Can you work these out from the model? Positions are in its coordinate system, mm. Coordinates: 2 decimals unless noted, no trailing zeros. Order: outer loops, then holes, each group sorted by start corner. A loop starts at its lowest first (then second) coordinate and runs counter-clockwise, first axis right, second up. Notation, with made-up numbers: (39, -6.75) -> (93, -6.75) arc R33 cw to (93, 26.25) -> close; hole circle Ø2 at (61.5, -33.5). An arc over 180 degrees is marked (long way). Answer as a JSON object with one key per item and string values. Group by question number.
(1) I want a section at A-A, the plane z = 0. List the corners of the cut face in (x, y) for me.
(2) I need wall thicknesses on line 1 (Y direction, x = 1.3, z = 0.1); line 2 (Y direction, x = 1.3, z = 0.7); line 3 (Z direction, x = -0.95, y = 3). Which ranges of each line are inside material? Lowest first, please.
(3) For pin 1 (1.5 mm diameter, centred on y = 56.5, z = 1, fed in from +X), with a flat end and sliding along its axis, tell me the tip position at first contact or that it passes through.
(4) I want a section at C-C, the plane y = 71.2. List the corners of the cut face in (x, z) for me (1 decimal), plus the area to 3 significant figures.
(5) I want a section at B-B, the plane y = 34.5. List the corners of the cut face in (x, z) for me (1 decimal), plus the area to 3 significant figures.
from build123d import *

# Parameters (mm, degrees)
SKETCH1_R                      = 1.5875
BOSS_EXTRUDE1_DEPTH            = 74.2
CUT_EXTRUDE1_REACH             = 3.587
SKETCH2_R                      = 1
CUT_EXTRUDE1_DIRECTION_2_REACH = 3.587


with BuildPart() as part:
    # Sketch1 → Boss-Extrude1 (new body)
    with BuildSketch(Plane(origin=(0, 0, 0), x_dir=(1, 0, 0), z_dir=(0, 1, 0))):
        Circle(SKETCH1_R)
    extrude(amount=BOSS_EXTRUDE1_DEPTH)

    # Sketch2 → Cut-Extrude1 (cut, up to next)
    with BuildSketch(Plane(origin=(0, 0, 0), x_dir=(0, 0, -1), z_dir=(1, 0, 0)), mode=Mode.PRIVATE) as cut_extrude1_sk1:
        with Locations((0, 71.2)):
            Circle(SKETCH2_R)
    cut_extrude1_tool1 = extrude(cut_extrude1_sk1.sketch, amount=-CUT_EXTRUDE1_REACH, mode=Mode.PRIVATE) & part.part
    add(cut_extrude1_tool1.solids().sort_by_distance((0, 71.2, 0))[0], mode=Mode.SUBTRACT)
    # Sketch2 → Cut-Extrude1 (cut, up to next)
    with BuildSketch(Plane(origin=(0, 0, 0), x_dir=(0, 0, -1), z_dir=(1, 0, 0)), mode=Mode.PRIVATE) as cut_extrude1_sk2:
        with Locations((0, 3)):
            Circle(SKETCH2_R)
    cut_extrude1_tool2 = extrude(cut_extrude1_sk2.sketch, amount=-CUT_EXTRUDE1_REACH, mode=Mode.PRIVATE) & part.part
    add(cut_extrude1_tool2.solids().sort_by_distance((0, 3, 0))[0], mode=Mode.SUBTRACT)

    # Sketch2 → Cut-Extrude1 direction 2 (cut, up to next)
    with BuildSketch(Plane(origin=(0, 0, 0), x_dir=(0, 0, -1), z_dir=(1, 0, 0)), mode=Mode.PRIVATE) as cut_extrude1_direction_2_sk1:
        with Locations((0, 71.2)):
            Circle(SKETCH2_R)
    cut_extrude1_direction_2_tool1 = extrude(cut_extrude1_direction_2_sk1.sketch, amount=CUT_EXTRUDE1_DIRECTION_2_REACH, mode=Mode.PRIVATE) & part.part
    add(cut_extrude1_direction_2_tool1.solids().sort_by_distance((0, 71.2, 0))[0], mode=Mode.SUBTRACT)
    # Sketch2 → Cut-Extrude1 direction 2 (cut, up to next)
    with BuildSketch(Plane(origin=(0, 0, 0), x_dir=(0, 0, -1), z_dir=(1, 0, 0)), mode=Mode.PRIVATE) as cut_extrude1_direction_2_sk2:
        with Locations((0, 3)):
            Circle(SKETCH2_R)
    cut_extrude1_direction_2_tool2 = extrude(cut_extrude1_direction_2_sk2.sketch, amount=CUT_EXTRUDE1_DIRECTION_2_REACH, mode=Mode.PRIVATE) & part.part
    add(cut_extrude1_direction_2_tool2.solids().sort_by_distance((0, 3, 0))[0], mode=Mode.SUBTRACT)


solid = part.part
Computed values:
{
 "1": {"outline": "(-1.59, 0) -> (1.59, 0) -> (1.59, 2) -> (-1.59, 2) -> close; (-1.59, 4) -> (1.59, 4) -> (1.59, 70.2) -> (-1.59, 70.2) -> close; (-1.59, 72.2) -> (1.59, 72.2) -> (1.59, 74.2) -> (-1.59, 74.2) -> close"},
 "2": {"line 1": "y = 0 to 2.01, 3.99 to 70.21, 72.19 to 74.2", "line 2": "y = 0 to 2.29, 3.71 to 70.49, 71.91 to 74.2", "line 3": "z = -1.27 to -1, 1 to 1.27"},
 "3": {"pin 1": "stops at x = 1.57"},
 "4": {"outline": "(-1.2, -1) arc R1.6 ccw to (1.2, -1) -> close; (-1.2, 1) -> (1.2, 1) arc R1.6 ccw to start", "area": "2.02 mm2"},
 "5": {"outline": "circle Ø3.2 at (0, 0)", "area": "7.92 mm2"}
}
